Work out the finished part from the listing and answer in its coordinate system (mm). A direction names the side the tool comes from. Round coordinates to 2 decimals unless told otherwise and drop trailing zeros. Write each loop counter-clockwise with the first axis right and the second up, starting at its lowest first coordinate (ties: lowest second). Pieces come first, ordered by that corner, then holes. Notation, with made-up numbers: (79, -7.75) -> (87, -7.75) arc R18 cw to (87, 19.25) -> close; hole circle Ø6 at (-28, 31.5). An arc over 180 degrees is marked (long way). One line per item, written item: value.
```python
from build123d import *

# Parameters (mm, degrees)
SKETCH1_W           = 30
SKETCH1_H           = 10
SKETCH1_R           = 2.555
BOSS_EXTRUDE1_DEPTH = 5
SKETCH2_R           = 1.25
CUT_EXTRUDE1_DEPTH  = 28.386127875
CUT_EXTRUDE2_START  = -5
SKETCH2_3_R         = 1.25
CUT_EXTRUDE2_DEPTH  = 5
FILLET1_R           = 5
FILLET2_R           = 1


# Some blends are built 0.0001 mm under size
with BuildPart() as part:
    # Sketch1 → Boss-Extrude1 (new body)
    with BuildSketch(Plane(origin=(0, 0, 0), x_dir=(1, 0, 0), z_dir=(0, 1, 0))):
        with Locations((10, 0)):
            Rectangle(SKETCH1_W, SKETCH1_H)
        with Locations(Location((0, 0, 0), (0, 0, 270))):
            Circle(SKETCH1_R, mode=Mode.SUBTRACT)
        with Locations(Location((10, 0, 0), (0, 0, 270))):
            Circle(SKETCH1_R, mode=Mode.SUBTRACT)
    extrude(amount=BOSS_EXTRUDE1_DEPTH)

    # Sketch2 → Cut-Extrude1 (cut, through all)
    with BuildSketch(Plane.XY.offset(5)):
        with Locations((17.5, 2.5)):
            Circle(SKETCH2_R)
    extrude(amount=-CUT_EXTRUDE1_DEPTH, mode=Mode.SUBTRACT)

    # Sketch2<3> → Cut-Extrude2 (cut)
    with BuildSketch(Plane.XY.offset(5).offset(CUT_EXTRUDE2_START)):
        Polygon((18.625, 4.448557159), (16.375, 4.448557159), (15.25, 2.5), (16.375, 0.551442841), (18.625, 0.551442841), (19.75, 2.5), align=None)
        with Locations((17.5, 2.5)):
            Circle(SKETCH2_3_R, mode=Mode.SUBTRACT)
    extrude(amount=-CUT_EXTRUDE2_DEPTH, mode=Mode.SUBTRACT)

    # Fillet1
    fillet1_edges = [part.edges().sort_by_distance(p)[0] for p in [
        (-5, 2.5, -5),
        (-5, 2.5, 5),
        (25, 2.5, -5),
        (25, 2.5, 5),
    ]]
    fillet(fillet1_edges, radius=FILLET1_R - 0.0001)  # a hair under: the kernel refuses the full size

    # Fillet2
    # the kernel refuses this fillet: 1 mm, written as the material it takes off along each edge
    with BuildSketch(Plane(origin=(-0.0001, 5, 0.0001), x_dir=(-1, 0, 0), z_dir=(0, 0, -1))) as fillet2_piece_1:
        with BuildLine():
            CenterArc((4.9999 - FILLET2_R, -FILLET2_R), FILLET2_R, 0, 90)
            Line((4.9999, -FILLET2_R), (4.9999, 0))
            Line((4.9999, 0), (4.9999 - FILLET2_R, 0))
        make_face()
    revolve(axis=Axis((-0.0001, 5, 0.0001), (0, 1, 0)), revolution_arc=90, mode=Mode.SUBTRACT)
    with BuildSketch(Plane(origin=(-0.0001, 5, -0.0001), x_dir=(0, 0, -1), z_dir=(1, 0, 0))) as fillet2_piece_2:
        with BuildLine():
            CenterArc((4.9999 - FILLET2_R, -FILLET2_R), FILLET2_R, 0, 90)
            Line((4.9999 - FILLET2_R, 0), (4.9999, 0))
            Line((4.9999, 0), (4.9999, -FILLET2_R))
        make_face()
    revolve(axis=Axis((-0.0001, 5, -0.0001), (0, 1, 0)), revolution_arc=90, mode=Mode.SUBTRACT)
    with BuildSketch(Plane(origin=(-0.0001, 5, -5), x_dir=(0, -1, 0), z_dir=(1, 0, 0))) as fillet2_piece_3:
        with BuildLine():
            CenterArc((FILLET2_R, -FILLET2_R), FILLET2_R, 90, 90)
            Line((0, -FILLET2_R), (0, 0))
            Line((0, 0), (FILLET2_R, 0))
        make_face()
    extrude(amount=20.0002, mode=Mode.SUBTRACT)
    with BuildSketch(Plane(origin=(20.0001, 5, -0.0001), x_dir=(0, 0, -1), z_dir=(-1, 0, 0))) as fillet2_piece_4:
        with BuildLine():
            CenterArc((4.9999 - FILLET2_R, FILLET2_R), FILLET2_R, 270, 90)
            Line((4.9999 - FILLET2_R, 0), (4.9999, 0))
            Line((4.9999, 0), (4.9999, FILLET2_R))
        make_face()
    revolve(axis=Axis((20.0001, 5, -0.0001), (0, -1, 0)), revolution_arc=90, mode=Mode.SUBTRACT)
    with BuildSketch(Plane(origin=(20.0001, 5, 0.0001), x_dir=(1, 0, 0), z_dir=(0, 0, -1))) as fillet2_piece_5:
        with BuildLine():
            CenterArc((4.9999 - FILLET2_R, FILLET2_R), FILLET2_R, 270, 90)
            Line((4.9999, FILLET2_R), (4.9999, 0))
            Line((4.9999, 0), (4.9999 - FILLET2_R, 0))
        make_face()
    revolve(axis=Axis((20.0001, 5, 0.0001), (0, -1, 0)), revolution_arc=90, mode=Mode.SUBTRACT)
    with BuildSketch(Plane(origin=(20.0001, 5, 5), x_dir=(0, 0, -1), z_dir=(-1, 0, 0))) as fillet2_piece_6:
        with BuildLine():
            CenterArc((FILLET2_R, FILLET2_R), FILLET2_R, 180, 90)
            Line((0, FILLET2_R), (0, 0))
            Line((0, 0), (FILLET2_R, 0))
        make_face()
    extrude(amount=20.0002, mode=Mode.SUBTRACT)
    with BuildSketch(Plane(origin=(25, 5, -0.0001), x_dir=(-1, 0, 0), z_dir=(0, 0, 1)), Plane(origin=(-5, 5, 0.0001), x_dir=(1, 0, 0), z_dir=(0, 0, -1))) as fillet2_piece_7:
        with BuildLine():
            CenterArc((FILLET2_R, FILLET2_R), FILLET2_R, 180, 90)
            Line((0, FILLET2_R), (0, 0))
            Line((0, 0), (FILLET2_R, 0))
        make_face()
    extrude(amount=0.0002, mode=Mode.SUBTRACT)


solid = part.part
```
(1) Find section A-A on x = 17.5. Give the vertices of the cut face in (y, z), plus the area to 3 significant figures.
Reported:
outline: (0, -5) -> (0.55, -5) -> (0.55, 0) -> (1.25, 0) -> (1.25, 5) -> (0, 5) -> close; (3.75, 0) -> (4.45, 0) -> (4.45, -4.89) arc R1 ccw to (5, -4) -> (5, 4) arc R1 ccw to (4, 5) -> (3.75, 5) -> close
area: 17.6 mm2
(2) Consider probe 1 along Y at (x, z) = (18, -1.25); probe 2 along X at (y, z) = (4.75, -1.25); probe 3 along X at (y, z) = (3.95, 0.25). Determine where each line is inside the solid, lowest interval first.
Reported:
probe 1: y = 0 to 0.55, 4.45 to 5
probe 2: x = -4.49 to -2.23, 2.23 to 7.77, 12.23 to 24.49
probe 3: x = -4.99 to -2.54, 2.54 to 7.46, 12.54 to 24.99
(3) For a pull along Y with two mould halves and no side action, classify faces 3 (the face through (10.14, 4.699, 4.715)), 4 (the face through (19.18, 1.51, -2.46)), 5 (the face through (-2.494, 2.465, -0.554)) as pulls with the +Y half, pulls with the -Y half, needs draft (parallel to the pull), parting line crosses it, or undercut.
Reported:
face 3: pulls with the +Y half
face 4: undercut
face 5: needs draft
(4) Find section B-B on z = -0.5. Give the number of separate pieces and of enclosed holes in the cut face, plus the area to 3 significant figures.
Reported:
separate pieces: 3
enclosed holes: 1
area: 86.1 mm2
(5) Find section C-C on x = 10. Give the vertices of the cut face in (y, z) (3 decimals).
Reported:
outline: (0, -5) -> (4, -5) arc R1 ccw to (5, -4) -> (5, -2.555) -> (0, -2.555) -> close; (0, 2.555) -> (5, 2.555) -> (5, 4) arc R1 ccw to (4, 5) -> (0, 5) -> close
(6) A tool of negligible diameter and unlimited length cuts with its end or side. For faces 1 (the face through (15.82, 3.49, -2.46)), 2 (the face through (13, 0, 0)), from which of +Z, -Z, +X, -X, +Y, -Y can it reach the whole face along a straight path? Write none if from no direction.
Reported:
face 1: -Z
face 2: +Z, -Z, +X, -X, -Y
(7) A flat-ended cylindrical pin translates along its axis: pin 1 Ø0.7 at (x, z) = (18, -2.5) entering from -Y. Find the tip coordinate at first contact, or state that the pin passes through.
Reported:
pin 1: stops at y = 0
